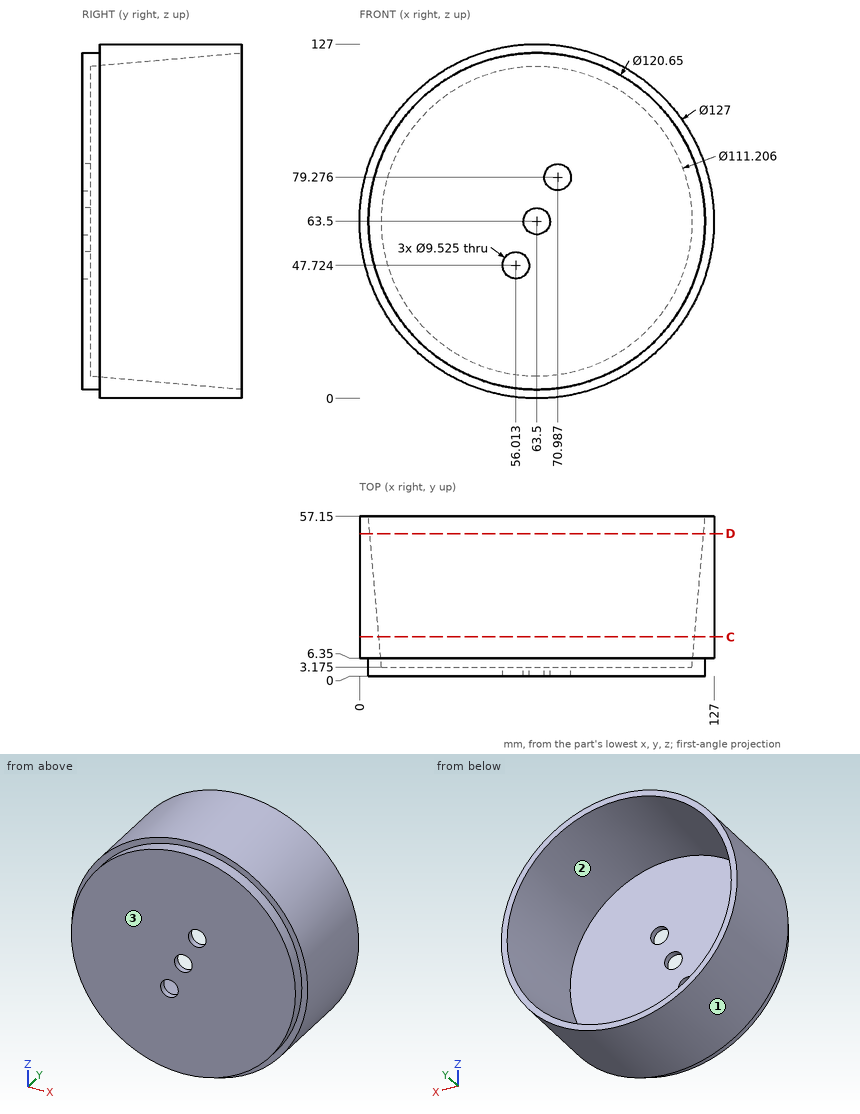
Can you work these out from the drawing? Everything is in mm from the part's minimum corner. Coordinates: 2 decimals unless noted, no trailing zeros. Order: outer loops, then holes, each group sorted by start corner. A loop starts at its lowest first (then second) coordinate and runs counter-clockwise, first axis right, second up. Notation, with made-up numbers: M -16,77 L -9,77 A18 ccw -9,88 Z; hole C -29,19.25 d10. An arc over 180 degrees is marked long. Answer as CSV lines item,"result". Start each with the question number.
1. We'd pull the mould along Z, two halves only. Please class the marked faces 1, 2 and 3: released by +Z, released by -Z, zero draft, split by the parting line, or undercut.
2. For pin 1 (4 mm diameter, centred on x = 60, y = 13.5, fed in from +Z); pin 2 (6 mm diameter, centred on y = 46, z = 114, fed in from +X); pin 3 (10 mm diameter, centred on y = 11, z = 30.5, fed in from +X); pin 4 (5.5 mm diameter, centred on x = 56.01, z = 47.72, fed in from -Y), each with a flat end and sliding along its axis, tell me the tip position at first contact or that it passes through.
3. I need wall thicknesses on line 1 (X direction, y = 1, z = 63); line 2 (Y direction, x = 77.5, z = 68) (1 decimal); line 3 (X direction, y = 10.5, z = 90) (1 decimal). Which ranges of each line are inside material? Lowest first, please. Write a range as [from, to].
4. I want a section at C-C, the plane y = 14. Write out the boundary of the cut face in (x, z), and give its area (3 significant figures).
5. I want a section at D-D, the plane y = 51. Write out the boundary of the cut face in (x, z), and give its area (3 significant figures).
Recorded:
1,face 1,"split by the parting line"
1,face 2,"undercut"
1,face 3,"zero draft"
2,pin 1,"stops at z = 126.98"
2,pin 2,"stops at x = 105.64"
2,pin 3,"stops at x = 120.49"
2,pin 4,"passes through"
3,line 1,"x = [3.18, 58.76], [68.24, 123.82]"
3,line 2,"y = [0, 3.2]"
3,line 3,"x = [5.8, 13.9], [113.1, 121.2]"
4,outline,"C 63.5,63.5 d127; hole C 63.5,63.5 d113.1"
4,area,"2,620 mm2"
5,outline,"C 63.5,63.5 d127; hole C 63.5,63.5 d119.57"
5,area,"1,440 mm2"
